Check sheet for the drawn part. Datum: minimum x, y, z corner. Units: mm. Round coordinates to 2 decimals unless told otherwise and drop trailing zeros. Write each loop counter-clockwise with the first axis right and the second up, starting at its lowest first coordinate (ties: lowest second). Pieces come first, ordered by that corner, then holes. Notation, with made-up numbers: M 6,37 L 11,37 A11 cw 11,54 Z; hole C -29.5,50.5 d6. An arc over 180 degrees is marked long. One line per item, written item: value. Start each with the question number.
1. Section check A-A (x = 112.5). Record the boundary of the cut face in (y, z), and give its area (3 significant figures).
2. Section check B-B (y = 112.5). Record the boundary of the cut face in (x, z), and give its area (3 significant figures).
3. Section check C-C (z = 7.25). Count the separate pieces of the cut face and the enclosed holes in it, and give its area (3 significant figures).
4. Scan lines: probe 1 along X at (y, z) = (112, 3) (1 decimal); probe 2 along Y at (x, z) = (111, 4.25); probe 3 along X at (y, z) = (61.5, 7) (1 decimal). Record each from-to range of solid material in increasing order. Write a range as [from, to].
5. Section check D-D (y = 88.5). Record the boundary of the cut face in (x, z), and give its area (3 significant figures).
6. Depth check by flat-ended pin: P1, Ø3, axis at y = 74.5, z = 3.5, coming from the -X side (1 decimal); P2, Ø20, axis at x = 181.27, y = 162.46, coming from the -Z side; P3, Ø1, axis at y = 27.5, z = 2, coming from the -X side; P4, Ø2, axis at y = 69, z = 7.5, coming from the +X side. Enter the tip coordinate at first touch or a pass-through.
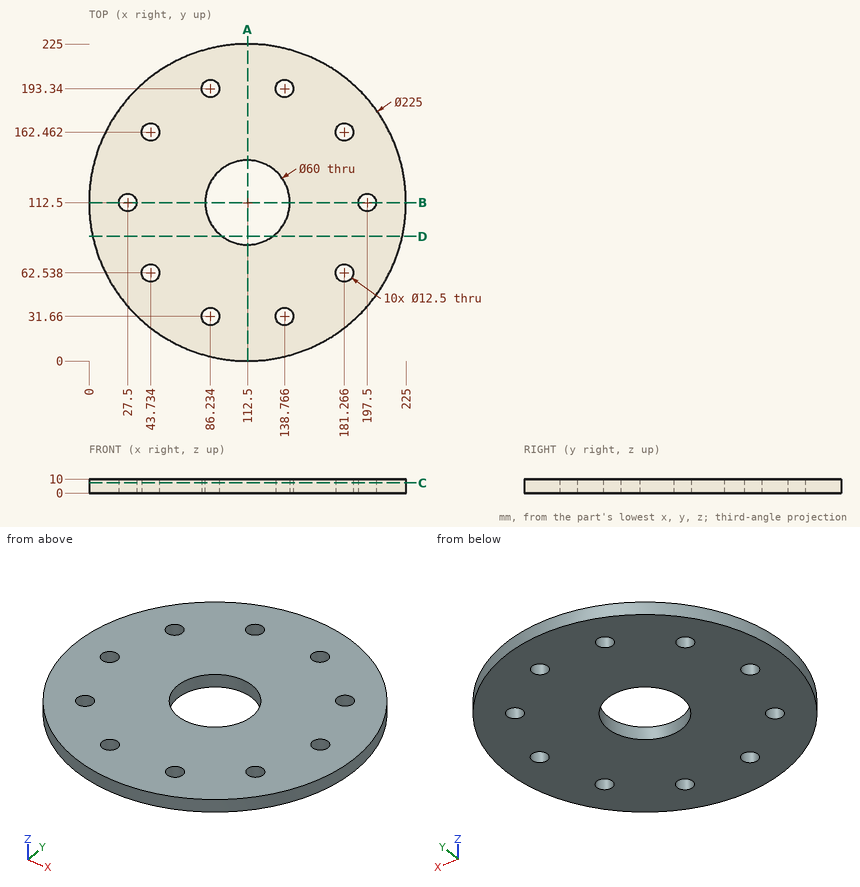
Result sheet:
1. outline: M 0,0 L 82.5,0 L 82.5,10 L 0,10 Z; M 142.5,0 L 225,0 L 225,10 L 142.5,10 Z
1. area: 1,650 mm2
2. outline: M 0,0 L 21.25,0 L 21.25,10 L 0,10 Z; M 33.75,0 L 82.5,0 L 82.5,10 L 33.75,10 Z; M 142.5,0 L 191.25,0 L 191.25,10 L 142.5,10 Z; M 203.75,0 L 225,0 L 225,10 L 203.75,10 Z
2. area: 1,400 mm2
3. separate pieces: 1
3. enclosed holes: 11
3. area: 35,700 mm2
4. probe 1: x = [0, 21.3], [33.7, 82.5], [142.5, 191.3], [203.7, 225]
4. probe 2: y = [0.01, 82.54], [142.46, 224.99]
4. probe 3: x = [12.2, 37.6], [49.9, 175.1], [187.4, 212.8]
5. outline: M 2.59,0 L 94.5,0 L 94.5,10 L 2.59,10 Z; M 130.5,0 L 222.41,0 L 222.41,10 L 130.5,10 Z
5. area: 1,840 mm2
6. P1: stops at x = 6.1
6. P2: stops at z = 0
6. P3: stops at x = 38.23
6. P4: stops at x = 216.66
